Here's how the part is built. I have some questions about the finished solid (model axes, mm). A direction names the side the tool comes from. Round coordinates to 2 decimals unless told otherwise and drop trailing zeros. Write each loop counter-clockwise with the first axis right and the second up, starting at its lowest first coordinate (ties: lowest second). Pieces come first, ordered by that corner, then holes. Notation, with made-up numbers: M -7,64 L 20,64 A32 ccw 20,97 Z; hole C 27.5,35 d3. An arc over 180 degrees is marked long. Write item = value, one per line. Start each with the question number.
(1) I need wall thicknesses on line 1 along X through (y, z) = (1.5, 1.5); line 2 along X through (y, z) = (4.75, 29); line 3 along Z through (x, y) = (-12.5, 3.25). Which ranges of each line are inside material? Lowest first, please.
(2) Will these pins go through, and if not, where does the flat tip stop? pin 1 Ø1.2 at (x, z) = (6.5, 25) entering from +Y; pin 2 Ø5 at (x, y) = (-14, 8) entering from +Z; pin 3 Ø2 at (y, z) = (8, 20.5) entering from -X.
(3) On a 3-axis mill with a long thin cutter (end or side, diameter ignored), from which of +Z, -Z, +X, -X, +Y, -Y can I reach the whole of each face in a straight line? I mean faces 5 (the flat face through (4.419, 3, 0)), 6 (the flat face through (-10.84, 8, 25)), 7 (the flat face through (-12.84, 10, 25)), 8 (the flat face through (-12, 8, 31.649)). Say none if no direction works.
(4) I want a section at C-C (z = -4.5). List the corners of the cut face in (x, y) for me.
(5) If we mould it in two halves opening along X, with no side actions, what happens to faces 1 (the cylindrical face through (-14.042, 6.141, 24.551)), 2 (the flat face through (-1, 3, 17.149)), 3 (the flat face through (-12, 8, 17.649)), 4 (the flat face through (-9.34, 3, 25))? For each: released by +X, released by -X, zero draft, split by the parting line, or undercut.
(6) I want a section at B-B (z = 27). List the corners of the cut face in (x, y) for me, and give its area (3 significant figures).
(7) I want a section at D-D (x = -20.5). List the corners of the cut face in (y, z) for me.
(8) I want a section at A-A (x = -2). List the corners of the cut face in (y, z) for me.
```python
from build123d import *

# Parameters (mm, degrees)
SKETCH1_W           = 50
SKETCH1_H           = 25
BOSS_EXTRUDE1_DEPTH = 5
SKETCH2_W           = 13.8
SKETCH2_H           = 15.8
CUT_EXTRUDE1_DEPTH  = 5
SKETCH3_W           = 14
SKETCH3_H           = 16.1
CUT_EXTRUDE2_DEPTH  = 5
SKETCH5_W           = 3
SKETCH5_H           = 1
SKETCH5_W_2         = 6
CUT_EXTRUDE3_DEPTH  = 1
SKETCH6_W           = 50
SKETCH6_H           = 25
BOSS_EXTRUDE2_DEPTH = 5
SKETCH7_W           = 16.25
SKETCH7_H           = 14.5
CUT_EXTRUDE4_DEPTH  = 4
SKETCH8_W           = 14.75
SKETCH8_H           = 14.5
CUT_EXTRUDE5_DEPTH  = 1
SKETCH9_W           = 2.5
SKETCH9_H           = 14
BOSS_EXTRUDE3_DEPTH = 4.6
SKETCH10_W          = 5
SKETCH10_H          = 14
BOSS_EXTRUDE4_DEPTH = 2.5
BOSS_EXTRUDE5_DEPTH = 14
FILLET1_R           = 1
SKETCH12_W          = 2
SKETCH12_H          = 14
BOSS_EXTRUDE6_DEPTH = 6
FILLET2_R           = 4
FILLET3_R           = 1
FILLET4_R           = 0.5


with BuildPart() as part:
    # Sketch1 → Boss-Extrude1 (new body)
    with BuildSketch(Plane(origin=(0, 0, 0), x_dir=(1, 0, 0), z_dir=(0, 1, 0))):
        Rectangle(SKETCH1_W, SKETCH1_H)
    extrude(amount=BOSS_EXTRUDE1_DEPTH)

    # Sketch2 → Cut-Extrude1 (cut)
    with BuildSketch(Plane(origin=(0, 5, 0), x_dir=(1, 0, 0), z_dir=(0, 1, 0))):
        with Locations((-12.471632497, -0.196290121)):
            Rectangle(SKETCH2_W, SKETCH2_H)
    extrude(amount=-CUT_EXTRUDE1_DEPTH, mode=Mode.SUBTRACT)

    # Sketch3 → Cut-Extrude2 (cut)
    with BuildSketch(Plane(origin=(0, 5, 0), x_dir=(1, 0, 0), z_dir=(0, 1, 0))):
        with Locations((11.418853314, -0.27633095)):
            Rectangle(SKETCH3_W, SKETCH3_H)
    extrude(amount=-CUT_EXTRUDE2_DEPTH, mode=Mode.SUBTRACT)

    # Sketch5 → Cut-Extrude3 (cut)
    with BuildSketch(Plane(origin=(0, 5, 0), x_dir=(1, 0, 0), z_dir=(0, 1, 0))):
        with Locations((-12.529830787, 10.403858803)):
            Rectangle(SKETCH5_W, SKETCH5_H)
        with Locations((12.528710417, 10.30293358)):
            Rectangle(SKETCH5_W_2, SKETCH5_H)
    extrude(amount=-CUT_EXTRUDE3_DEPTH, mode=Mode.SUBTRACT)

    # Sketch6 → Boss-Extrude2 (add)
    with BuildSketch(Plane(origin=(0, 0, 0), x_dir=(1, 0, 0), z_dir=(0, 1, 0))):
        with Locations((0, -25)):
            Rectangle(SKETCH6_W, SKETCH6_H)
    extrude(amount=BOSS_EXTRUDE2_DEPTH)

    # Sketch7 → Cut-Extrude4 (cut)
    with BuildSketch(Plane(origin=(0, 5, 0), x_dir=(1, 0, 0), z_dir=(0, 1, 0))):
        with Locations((-1.214601825, -24.398968546)):
            Rectangle(SKETCH7_W, SKETCH7_H)
    extrude(amount=-CUT_EXTRUDE4_DEPTH, mode=Mode.SUBTRACT)

    # Sketch8 → Cut-Extrude5 (cut)
    with BuildSketch(Plane(origin=(0, 1, 0), x_dir=(1, 0, 0), z_dir=(0, 1, 0))):
        with Locations((-1.964601825, -24.398968546)):
            Rectangle(SKETCH8_W, SKETCH8_H)
    extrude(amount=-CUT_EXTRUDE5_DEPTH, mode=Mode.SUBTRACT)

    # Sketch9 → Boss-Extrude3 (add)
    with BuildSketch(Plane(origin=(0, 5, 0), x_dir=(1, 0, 0), z_dir=(0, 1, 0))):
        with Locations((13.660398175, -24.242407708)):
            Rectangle(SKETCH9_W, SKETCH9_H)
    extrude(amount=BOSS_EXTRUDE3_DEPTH)

    # Sketch10 → Boss-Extrude4 (add)
    with BuildSketch(Plane(origin=(0, 9.6, 0), x_dir=(1, 0, 0), z_dir=(0, 1, 0))):
        with Locations((12.410398175, -24.242407708)):
            Rectangle(SKETCH10_W, SKETCH10_H)
    extrude(amount=BOSS_EXTRUDE4_DEPTH)

    # Sketch11 → Boss-Extrude5 (add)
    with BuildSketch(Plane.XY.offset(31.242407708)):
        Polygon((14.910398175, 5), (18.418853314, 5), (14.910398175, 12.1), align=None)
    extrude(amount=-BOSS_EXTRUDE5_DEPTH)

    # Fillet1
    fillet1_edges = [part.edges().sort_by_distance(p)[0] for p in [
        (14.910398175, 12.1, 24.242407708),
        (18.418853314, 5, 24.242407708),
    ]]
    fillet(fillet1_edges, radius=FILLET1_R)

    # Sketch12 → Boss-Extrude6 (add)
    with BuildSketch(Plane(origin=(0, 5, 0), x_dir=(1, 0, 0), z_dir=(0, 1, 0))):
        with Locations((-11.839601825, -24.648968546)):
            Rectangle(SKETCH12_W, SKETCH12_H)
    extrude(amount=BOSS_EXTRUDE6_DEPTH)

    # Fillet2
    fillet2_edges = [part.edges().sort_by_distance(p)[0] for p in [
        (-12.839601825, 5, 24.648968546),
    ]]
    fillet(fillet2_edges, radius=FILLET2_R)

    # Fillet3
    fillet3_edges = [part.edges().sort_by_distance(p)[0] for p in [
        (12.410398175, 5, 24.242407708),
    ]]
    fillet(fillet3_edges, radius=FILLET3_R)

    # Fillet4
    fillet4_edges = [part.edges().sort_by_distance(p)[0] for p in [
        (-10.839601825, 5, 24.648968546),
    ]]
    fillet(fillet4_edges, radius=FILLET4_R)


solid = part.part
```
Returned:
q1.line_1 = -25 to -19.37, -5.57 to 4.42, 18.42 to 25
q1.line_2 = -25 to -9.34, 6.91 to 25
q1.line_3 = -12.5 to -7.7, 8.1 to 37.5
q2.pin_1 = 5
q2.pin_2 = 31.65
q2.pin_3 = -13.38
q3.face_5 = +Y, -Y
q3.face_6 = +Z, -Z, +Y
q3.face_7 = +Z, -Z, -X, +Y
q3.face_8 = +Z, +X, -X, +Y
q4.outline = M -25,0 L -19.37,0 L -19.37,5 L -25,5 Z; M -5.57,0 L 4.42,0 L 4.42,5 L -5.57,5 Z; M 18.42,0 L 25,0 L 25,5 L 18.42,5 Z
q5.face_1 = released by -X
q5.face_2 = undercut
q5.face_3 = zero draft
q5.face_4 = undercut
q6.outline = M -25,0 L -9.34,0 L -9.34,5 L -10.34,5 A0.5 cw -10.84,5.5 L -10.84,11 L -12.84,11 L -12.84,9 A4 cw -16.84,5 L -25,5 Z; M 5.41,0 L 25,0 L 25,5 L 19.04,5 A1 cw 18.14,5.56 L 15.19,11.54 A1 ccw 14.29,12.1 L 9.91,12.1 L 9.91,9.6 L 12.41,9.6 L 12.41,6 A1 cw 11.41,5 L 6.91,5 L 6.91,1 L 5.41,1 Z
q6.area = 222 mm²
q7.outline = M 0,-12.5 L 5,-12.5 L 5,37.5 L 0,37.5 Z
q8.outline = M 0,-12.5 L 5,-12.5 L 5,17.15 L 0,17.15 Z; M 0,31.65 L 5,31.65 L 5,37.5 L 0,37.5 Z
